Could you check a few things on this model? Use its own coordinates, in mm. Face numbers are marked on the shaded views. Give positions to 0.01 mm unless a question says otherwise; leave off trailing zeros. Write each loop counter-clockwise with the first axis right and the second up, starting at its lowest first coordinate (ties: lowest second). Pieces come first, ordered by that corner, then holes. Notation, with made-up numbers: M 35.5,19 L 71.5,19 A27 cw 71.5,42 Z; hole C -24.75,58 d3. An arc over 180 degrees is marked long. Write each question's results on one line, items separated by ' | '. Start each with the question number.
Autodesk Inventor part; units mm, degrees
ref_plane "YZ Plane" through (0, 0, 0) normal (1, 0, 0) x (0, 1, 0)
ref_plane "XZ Plane" through (0, 0, 0) normal (0, 1, 0) x (-1, 0, 0)
ref_plane "XY Plane" through (0, 0, 0) normal (0, 0, 1) x (1, 0, 0)
sketch "Sketch9" plane through (0, 0, 0) normal (0, 1, 0) x (-1, 0, 0)
  line L0 (15, 15) -> (-15, 15)
  line L1 (-15, 15) -> (-15, -15)
  line L2 (-15, -15) -> (15, -15)
  line L3 (15, -15) -> (15, 15)
  line L4 (15, 15) -> (-15, -15) construction
  line L5 (-15, 15) -> (15, -15) construction
  line L6 (-13, 13) -> (13, 13)
  line L7 (13, 13) -> (13, -13)
  line L8 (13, -13) -> (-13, -13)
  line L9 (-13, -13) -> (-13, 13)
  point P0 (0, 0)
  dimension "d172" = 30
  dimension "d173" = 30
  dimension "d174" = 2
extrude "Extrusion3" add sketch "Sketch9" against normal blind 450
sketch "Sketch10" plane through (0, 0, 0) normal (1, 0, 0) x (0, 1, 0)
  line L0 (0, 15) -> (0, -15) construction
  line L1 (0, 15) -> (-450, 15) construction
  line L2 (-450, -15) -> (-450, 15) construction
  line L3 (0, -15) -> (-450, -15) construction
  line L4 (-68.5, 8.5) -> (-51.5, 8.5)
  line L5 (-51.5, 8.5) -> (-51.5, -8.5)
  line L6 (-51.5, -8.5) -> (-68.5, -8.5)
  line L7 (-68.5, -8.5) -> (-68.5, 8.5)
  line L8 (-68.5, 8.5) -> (-51.5, -8.5) construction
  line L9 (-51.5, 8.5) -> (-68.5, -8.5) construction
  line L10 (-268.5, 8.5) -> (-251.5, 8.5)
  line L11 (-251.5, 8.5) -> (-251.5, -8.5)
  line L12 (-251.5, -8.5) -> (-268.5, -8.5)
  line L13 (-268.5, -8.5) -> (-268.5, 8.5)
  line L14 (-268.5, 8.5) -> (-251.5, -8.5) construction
  line L15 (-251.5, 8.5) -> (-268.5, -8.5) construction
  line L16 (-428.5, 8.5) -> (-411.5, 8.5)
  line L17 (-411.5, 8.5) -> (-411.5, -8.5)
  line L18 (-411.5, -8.5) -> (-428.5, -8.5)
  line L19 (-428.5, -8.5) -> (-428.5, 8.5)
  line L20 (-428.5, 8.5) -> (-411.5, -8.5) construction
  line L21 (-411.5, 8.5) -> (-428.5, -8.5) construction
  circle A0 centre (-470, 0) radius 8.5
  line L22 (0, 0) -> (30, 0)
  circle A1 centre (-60, 0) radius 8.5
  circle A2 centre (-260, 0) radius 8.5
  circle A3 centre (-420, 0) radius 8.5
  dimension "d177" = 17
  dimension "d178" = 17
  dimension "d181" = 30
  dimension "d182" = 90
  dimension "d183" = 290
  dimension "d184" = 450
  dimension "d185" = 500
  dimension "d186" = 17
extrude "Extrusion4" cut sketch "Sketch10" along normal through all contours A1 | A2 | A3
properties part number "PNS 755 FDS 1200 way tube 2" material "Stainless Steel"
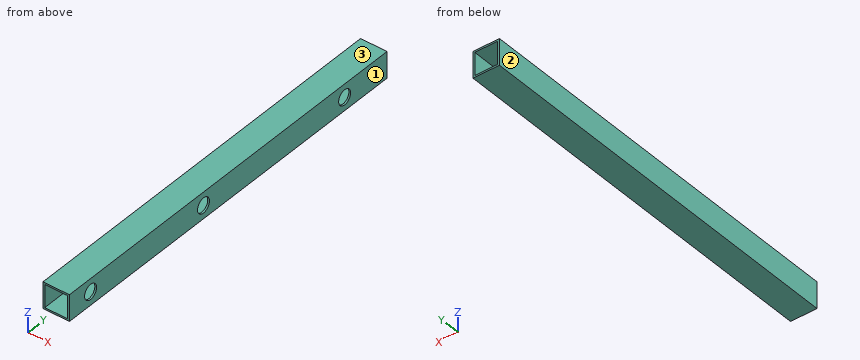
Q1. If we section it at B-B (z = 0): Please give me the cut outline in (x, y).
Q2. If we section it at C-C (y = -179): Please give me the cut outline in (x, z), plus the area to 3 significant figures.
Q3. Please list where these lines run through material, in increasing order: line 1 (Y direction, x = 13.5, z = 0); line 2 (Z direction, x = 9.25, y = -253). Write a range as [from, to].
Q4. If we section it at D-D (y = -420): Please give me the cut outline in (x, z), plus the area to 3 significant figures.
Q5. If we mould it in two halves opening along X, with no side actions, what happens to the marked faces 1, 2 and 3? For each: pulls with the +X half, pulls with the -X half, needs draft (parallel to the pull), parting line crosses it, or undercut.
Q6. If we section it at A-A (x = -0.25): Please give me the cut outline in (y, z), plus the area to 3 significant figures.
Determined:
1) outline: M -15,-450 L -13,-450 L -13,0 L -15,0 Z; M 13,-450 L 15,-450 L 15,-428.5 L 13,-428.5 Z; M 13,-411.5 L 15,-411.5 L 15,-268.5 L 13,-268.5 Z; M 13,-251.5 L 15,-251.5 L 15,-68.5 L 13,-68.5 Z; M 13,-51.5 L 15,-51.5 L 15,0 L 13,0 Z
2) outline: M -15,-15 L 15,-15 L 15,15 L -15,15 Z; hole M -13,-13 L 13,-13 L 13,13 L -13,13 Z | area: 224 mm²
3) line 1: y = [-450, -428.5], [-411.5, -268.5], [-251.5, -68.5], [-51.5, 0] | line 2: z = [-15, -13], [13, 15]
4) outline: M -15,-15 L 15,-15 L 15,-8.5 L 13,-8.5 L 13,-13 L -13,-13 L -13,13 L 13,13 L 13,8.5 L 15,8.5 L 15,15 L -15,15 Z | area: 190 mm²
5) face 1: pulls with the +X half | face 2: pulls with the -X half | face 3: needs draft
6) outline: M -450,-15 L 0,-15 L 0,-13 L -450,-13 Z; M -450,13 L 0,13 L 0,15 L -450,15 Z | area: 1,800 mm²
